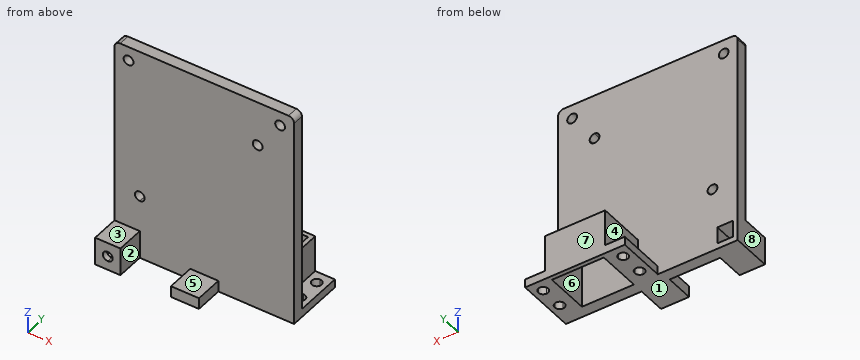
```python
from build123d import *

# Parameters (mm, degrees)
F0_W      = 64
F0_H      = 77
F1_DEPTH  = 4
F2_R      = 1.75
F3_DEPTH  = 25
F5_DEPTH  = 10
F7_DEPTH  = 25
F8_W      = 21.5
F8_H      = 16
F9_DEPTH  = 17
F10_W     = 18.5
F10_H     = 15.5
F11_DEPTH = 25
F12_W     = 17
F12_H     = 3
F13_DEPTH = 7
F14_W     = 17
F14_H     = 3
F15_DEPTH = 7
F17_DEPTH = 25
F19_DEPTH = 25
F21_DEPTH = 10
F22_DEPTH = 25
F23_W     = 5.5
F23_H     = 6
F23_R     = 1.75
F24_DEPTH = 12
F25_R     = 2


# Not quite as in the source:
# - a feature names something its author has since deleted; it is built from what else it names


with BuildPart() as f1:
    # F0 (on Front) → F1 (new body)
    with BuildSketch(Plane.XZ):
        Rectangle(F0_W, F0_H)
    extrude(amount=F1_DEPTH)

    # F2 (on face) → F3 (cut)
    with BuildSketch(Plane.XZ.offset(4)):
        with BuildLine():
            ThreePointArc((-28.75, 33.5), (-27, 31.75), (-25.25, 33.5))
            ThreePointArc((-25.25, 33.5), (-27, 35.25), (-28.75, 33.5))
        make_face()
        with Locations((27, 33.5)):
            Circle(F2_R)
    extrude(amount=-F3_DEPTH, mode=Mode.SUBTRACT)

    # F4 (on face) → F5 (join)
    with BuildSketch(Plane.XZ.offset(4)):
        Polygon((-5, -34.5), (-5, -38.5), (0, -38.5), (5, -38.5), (5, -34.5), align=None)
    extrude(amount=F5_DEPTH)

    # F6 (on face) → F7 (cut)
    with BuildSketch(Plane.XZ.offset(4)):
        with BuildLine():
            Line((19, 22.5), (19, 24.25))
            ThreePointArc((19, 24.25), (17.7625631329, 21.2625631329), (20.75, 22.5))
            Line((20.75, 22.5), (19, 22.5))
        make_face()
        with BuildLine():
            ThreePointArc((20.75, 22.5), (20.2374368671, 23.7374368671), (19, 24.25))
            Line((19, 24.25), (19, 22.5))
            Line((19, 22.5), (20.75, 22.5))
        make_face()
        with BuildLine():
            ThreePointArc((-21.25, -15.5), (-24.2374368671, -14.2625631329), (-23, -17.25))
            ThreePointArc((-23, -17.25), (-21.7625631329, -16.7374368671), (-21.25, -15.5))
        make_face()
    extrude(amount=-F7_DEPTH, mode=Mode.SUBTRACT)

    # F8 (on face) → F9 (join)
    with BuildSketch(Plane(origin=(0, 0, 0), x_dir=(-1, 0, 0), z_dir=(0, 1, 0))):
        with Locations((-14.25, -30.5)):
            Rectangle(F8_W, F8_H)
    extrude(amount=F9_DEPTH)

    # F10 (on face) → F11 (cut)
    with BuildSketch(Plane.XY.offset(-22.5)):
        with Locations((14.25, 7.75)):
            Rectangle(F10_W, F10_H)
    extrude(amount=-F11_DEPTH, mode=Mode.SUBTRACT)

    # F12 (on face) → F13 (join)
    with BuildSketch(Plane.YZ.offset(25)):
        with Locations((8.5, -37)):
            Rectangle(F12_W, F12_H)
    extrude(amount=F13_DEPTH)

    # F14 (on face) → F15 (join)
    with BuildSketch(Plane(origin=(3.5, 0, 0), x_dir=(0, -1, 0), z_dir=(-1, 0, 0))):
        with Locations((-8.5, -37)):
            Rectangle(F14_W, F14_H)
    extrude(amount=F15_DEPTH)

    # F16 (on face) → F17 (cut)
    with BuildSketch(Plane.XY.offset(-35.5)):
        with BuildLine():
            Line((0, 14.5), (0, 11))
            ThreePointArc((0, 11), (1.2374368671, 11.5125631329), (1.75, 12.75))
            ThreePointArc((1.75, 12.75), (1.2374368671, 13.9874368671), (0, 14.5))
        make_face()
        with BuildLine():
            ThreePointArc((0, 14.5), (-1.75, 12.75), (0, 11))
            Line((0, 11), (0, 14.5))
        make_face()
        with BuildLine():
            ThreePointArc((0, 6), (-1.75, 4.25), (0, 2.5))
            Line((0, 2.5), (0, 6))
        make_face()
        with BuildLine():
            Line((0, 6), (0, 2.5))
            ThreePointArc((0, 2.5), (1.2374368671, 3.0125631329), (1.75, 4.25))
            ThreePointArc((1.75, 4.25), (1.2374368671, 5.4874368671), (0, 6))
        make_face()
    extrude(amount=-F17_DEPTH, mode=Mode.SUBTRACT)

    # F18 (on face) → F19 (cut)
    with BuildSketch(Plane.XY.offset(-35.5)):
        with BuildLine():
            ThreePointArc((30.25, 12.75), (29.7374368671, 13.9874368671), (28.5, 14.5))
            Line((28.5, 14.5), (28.5, 11))
            ThreePointArc((28.5, 11), (29.7374368671, 11.5125631329), (30.25, 12.75))
        make_face()
        with BuildLine():
            ThreePointArc((30.25, 4.25), (29.7374368671, 5.4874368671), (28.5, 6))
            Line((28.5, 6), (28.5, 2.5))
            ThreePointArc((28.5, 2.5), (29.7374368671, 3.0125631329), (30.25, 4.25))
        make_face()
        with BuildLine():
            Line((28.5, 2.5), (28.5, 6))
            ThreePointArc((28.5, 6), (26.75, 4.25), (28.5, 2.5))
        make_face()
        with BuildLine():
            Line((28.5, 11), (28.5, 14.5))
            ThreePointArc((28.5, 14.5), (26.75, 12.75), (28.5, 11))
        make_face()
    extrude(amount=-F19_DEPTH, mode=Mode.SUBTRACT)

    # F20 (on face) → F21 (join)
    with BuildSketch(Plane.XZ.offset(4)):
        Polygon((-32, -28.5), (-32, -38.5), (-27.5, -38.5), (-23, -38.5), (-23, -28.5), align=None)
        with BuildLine():
            ThreePointArc((-25.75, -33.5), (-26.2625631329, -34.7374368671), (-27.5, -35.25))
            ThreePointArc((-27.5, -35.25), (-28.7374368671, -32.2625631329), (-25.75, -33.5))
        make_face(mode=Mode.SUBTRACT)
    extrude(amount=F21_DEPTH)

    # F22 (cut): a face of the model
    f22_faces = [f1.faces().sort_by_distance(p)[0] for p in [
        (-27.5, -4, -33.5),
    ]]
    extrude(f22_faces, amount=-F22_DEPTH, mode=Mode.SUBTRACT)

    # F23 (on face) → F24 (cut)
    with BuildSketch(Plane(origin=(0, 0, 0), x_dir=(-1, 0, 0), z_dir=(0, 1, 0))):
        with Locations((27.5, -33.5)):
            Rectangle(F23_W, F23_H)
        with Locations((27.5, -33.5)):
            Circle(F23_R, mode=Mode.SUBTRACT)
    extrude(amount=-F24_DEPTH, mode=Mode.SUBTRACT)

    # F25
    f25_edges = [f1.edges().sort_by_distance(p)[0] for p in [
        (-32, -2, 38.5),
        (32, -2, 38.5),
    ]]
    fillet(f25_edges, radius=F25_R)


solid = f1.part
```
Part model, mm, in its own coordinate system. Face numbers are marked on the shaded views. A direction names the side the tool comes from. Coordinates: 2 decimals unless noted, no trailing zeros. Order: outer loops, then holes, each group sorted by start corner. A loop starts at its lowest first (then second) coordinate and runs counter-clockwise, first axis right, second up. Notation, with made-up numbers: (89.25, 49.25) -> (142.25, 49.25) arc R10 ccw to (142.25, 56.25) -> close; hole circle Ø7 at (67, 60). An arc over 180 degrees is marked (long way). Put each result on its own line as item: value. Start each with the question number.
(1) Which spindle directions (+Z, -Z, +X, -X, +Y, -Y) get a long thin tool onto all of the face, cutting with end or side? Do the marked faces 1, 2, 3, 4 and 5. Say none if no direction does.
(2) Band-saw the part on B-B (y = -6). Give the cut face in (x, z), then the cut area to 3 significant figures.
(3) Probe line 1 along Y through (x, z) = (9.5, -27); line 2 along Z through (x, y) = (19, -2); line 3 along Z through (x, y) = (-23, -2.8). List the from-to ranges inside material, lowest first. Write a range as [from, to].
(4) Mould opens along X. For the marked faces 6, 7 and 8 say: pulls with the +X half, pulls with the -X half, needs draft (parallel to the pull), parting line crosses it, or undercut.
(5) Pin check, flat tips, straight feed: pin 1 Ø1.6 at (x, z) = (-26.5, -34) entering from +Y; pin 2 Ø8 at (y, z) = (8, -30.5) entering from -X; pin 3 Ø10 at (y, z) = (-10.5, -16.5) entering from +X; pin 4 Ø4.5 at (x, y) = (-26, -10.5) entering from +Z. Stop position of each tip, or through.
(6) Band-saw the part on A-A (z = -25.5). Give the cut face in (x, y).
(7) Band-saw the part on C-C (x = -17). Give the cut face in (y, z).
Determined:
1. face 1: -Z, +X, -X, +Y, -Y
1. face 2: +Z, -Z, -Y
1. face 3: +Z, +X, -X, -Y
1. face 4: +Z, -X, +Y
1. face 5: +Z, +X, -Y
2. outline: (-32, -38.5) -> (-23, -38.5) -> (-23, -28.5) -> (-32, -28.5) -> close; (-5, -38.5) -> (5, -38.5) -> (5, -34.5) -> (-5, -34.5) -> close; hole (-30.25, -36.5) -> (-24.75, -36.5) -> (-24.75, -30.5) -> (-30.25, -30.5) -> close
2. area: 97.0 mm²
3. line 1: y = [-4, 0], [15.5, 17]
3. line 2: z = [-38.5, 20.75], [24.25, 38.5]
3. line 3: z = [-38.5, -17.25], [-13.75, 38.5]
4. face 6: undercut
4. face 7: needs draft
4. face 8: pulls with the -X half
5. pin 1: stops at y = -12
5. pin 2: stops at x = 3.5
5. pin 3: passes through
5. pin 4: stops at z = -28.5
6. outline: (-32, -4) -> (32, -4) -> (32, 0) -> (25, 0) -> (25, 17) -> (3.5, 17) -> (3.5, 0) -> (-32, 0) -> close; hole (5, 0) -> (23.5, 0) -> (23.5, 15.5) -> (5, 15.5) -> close
7. outline: (-4, -38.5) -> (0, -38.5) -> (0, 38.5) -> (-4, 38.5) -> close
